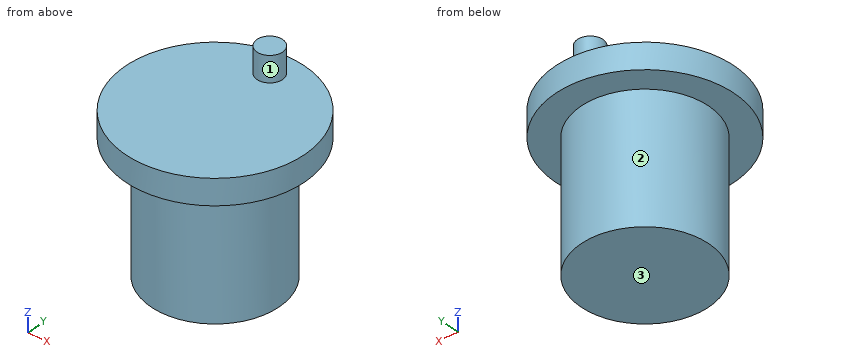
from build123d import *

# Parameters (mm, degrees)
SKETCH1_R           = 7
BOSS_EXTRUDE1_DEPTH = 2
SKETCH2_R           = 1
BOSS_EXTRUDE2_DEPTH = 2
SKETCH3_R           = 5
BOSS_EXTRUDE3_DEPTH = 10


with BuildPart() as part:
    # Sketch1 → Boss-Extrude1 (new body)
    with BuildSketch(Plane.XY):
        Circle(SKETCH1_R)
    extrude(amount=-BOSS_EXTRUDE1_DEPTH)

    # Sketch2 → Boss-Extrude2 (add)
    with BuildSketch(Plane.XY):
        with Locations((0, 5)):
            Circle(SKETCH2_R)
    extrude(amount=BOSS_EXTRUDE2_DEPTH)

    # Sketch3 → Boss-Extrude3 (add)
    with BuildSketch(Plane(origin=(0, 0, -2), x_dir=(-1, 0, 0), z_dir=(0, 0, -1))):
        Circle(SKETCH3_R)
    extrude(amount=BOSS_EXTRUDE3_DEPTH)


solid = part.part
Work out the finished part from the listing and answer in its coordinate system (mm). Face numbers are marked on the shaded views. A direction names the side the tool comes from. Give positions to 0.01 mm unless a question says otherwise; leave off trailing zeros. Order: outer loops, then holes, each group sorted by start corner. A loop starts at its lowest first (then second) coordinate and runs counter-clockwise, first axis right, second up. Notation, with made-up numbers: (22.25, -7) -> (31.25, -7) arc R19 ccw to (31.25, 3) -> close; hole circle Ø7 at (79, 87). An arc over 180 degrees is marked (long way). Answer as a JSON object with one key per item and string values. Group by question number.
1. Consider line 1 along Z through (x, y) = (-0.5, -1.5); line 2 along Z through (x, y) = (-0.25, 6); line 3 along X through (y, z) = (4, -0.5). Determine where each line is inside the solid, lowest interval first. Write a range as [from, to].
2. Flat-ended cylindrical pins translate along their axes: pin 1 Ø5 at (y, z) = (-2.5, -8) entering from +X; pin 2 Ø6 at (y, z) = (2, -0.5) entering from -X; pin 3 Ø5 at (x, y) = (-3.5, 3.5) entering from +Z; pin 4 Ø1.5 at (y, z) = (-1.5, -7.5) entering from -X. Find the tip coordinate at first contact, or state that the pin passes through.
3. Section A-A on y = 0 is taken. Determine the outline of the cut face in (x, z), plus the area to 3 significant figures.
4. Section C-C on z = -2.25 is taken. Determine the outline of the cut face in (x, y).
5. A tool of negligible diameter and unlimited length cuts with its end or side. For the marked faces 1, 2 and 3, from which of +Z, -Z, +X, -X, +Y, -Y can it reach the whole face along a straight path? Write none if from no direction.
6. Section B-B on x = -0.5 is taken. Determine the outline of the cut face in (y, z).
7. Section D-D on y = -3 is taken. Determine the outline of the cut face in (x, z).
Result sheet:
{
 "1": {"line 1": "z = [-12, 0]", "line 2": "z = [-2, 0]", "line 3": "x = [-5.74, 5.74]"},
 "2": {"pin 1": "stops at x = 5", "pin 2": "stops at x = -7", "pin 3": "stops at z = 0", "pin 4": "stops at x = -4.94"},
 "3": {"outline": "(-7, -2) -> (-5, -2) -> (-5, -12) -> (5, -12) -> (5, -2) -> (7, -2) -> (7, 0) -> (-7, 0) -> close", "area": "128 mm^2"},
 "4": {"outline": "circle Ø10 at (0, 0)"},
 "5": {"face 1": "+Z", "face 2": "-Z", "face 3": "-Z, +X, -X, +Y, -Y"},
 "6": {"outline": "(-6.98, -2) -> (-4.97, -2) -> (-4.97, -12) -> (4.97, -12) -> (4.97, -2) -> (6.98, -2) -> (6.98, 0) -> (5.87, 0) -> (5.87, 2) -> (4.13, 2) -> (4.13, 0) -> (-6.98, 0) -> close"},
 "7": {"outline": "(-6.32, -2) -> (-4, -2) -> (-4, -12) -> (4, -12) -> (4, -2) -> (6.32, -2) -> (6.32, 0) -> (-6.32, 0) -> close"}
}
